Source: CAD feature listing. Evaluate the final solid. Frame: model axes, mm. Face numbers are marked on the shaded views. A direction names the side the tool comes from. Round coordinates to 2 decimals unless told otherwise and drop trailing zeros. Order: outer loops, then holes, each group sorted by start corner. A loop starts at its lowest first (then second) coordinate and runs counter-clockwise, first axis right, second up.
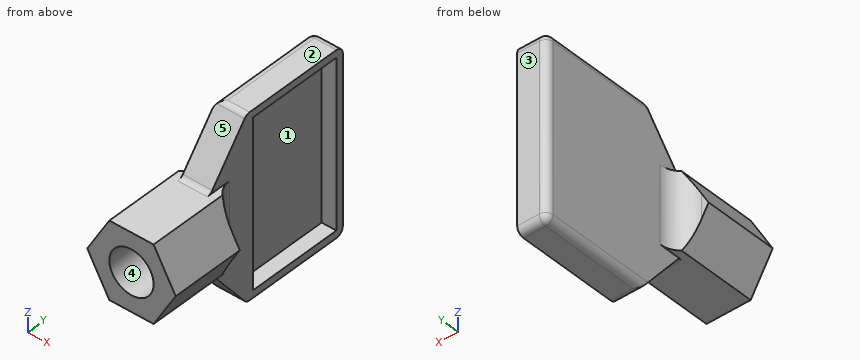
```python
from build123d import *

# Parameters (mm, degrees)
BOSS_EXTRUDE1_DEPTH      = 10
SKETCH2_R                = 3
CUT_EXTRUDE1_DEPTH       = 8
BOSS_EXTRUDE2_DEPTH      = 2
BOSS_EXTRUDE2_DEPTH_BACK = 2
SKETCH4_W                = 22.6
SKETCH4_H                = 13
CUT_EXTRUDE3_DEPTH       = 2
FILLET1_R                = 1
FILLET2_R                = 3


with BuildPart() as part:
    # Sketch1 → Boss-Extrude1 (new body)
    with BuildSketch(Plane(origin=(0, 0, 0), x_dir=(1, 0, 0), z_dir=(0, 1, 0))):
        Polygon((6, 0), (3, 5.196152423), (-3, 5.196152423), (-6, 0), (-3, -5.196152423), (3, -5.196152423), align=None)
    extrude(amount=BOSS_EXTRUDE1_DEPTH)

    # Sketch2 → Cut-Extrude1 (cut)
    with BuildSketch(Plane.XZ):
        with Locations(Location((0, 0, 0), (0, 0, 270))):
            Circle(SKETCH2_R)
    extrude(amount=-CUT_EXTRUDE1_DEPTH, mode=Mode.SUBTRACT)

    # Sketch3 → Boss-Extrude2 (add, two sides: drawn at the far end of the back side and taken through both)
    with BuildSketch(Plane(origin=(0, 0, 0), x_dir=(0, 0, -1), z_dir=(1, 0, 0)).offset(-BOSS_EXTRUDE2_DEPTH_BACK)):
        Polygon((0, 10), (5.196152423, 10), (12.3, 15.651732035), (12.3, 30.651732035), (0, 30.651732035), align=None)
        Polygon((-5.196152423, 10), (0, 10), (0, 30.651732035), (-12.3, 30.651732035), (-12.3, 15.651732035), align=None)
    extrude(amount=BOSS_EXTRUDE2_DEPTH + BOSS_EXTRUDE2_DEPTH_BACK)

    # Sketch4 → Cut-Extrude3 (cut)
    with BuildSketch(Plane(origin=(2, 0, 0), x_dir=(0, 0, -1), z_dir=(1, 0, 0))):
        with Locations((0, 23.151732035)):
            Rectangle(SKETCH4_W, SKETCH4_H)
    extrude(amount=-CUT_EXTRUDE3_DEPTH, mode=Mode.SUBTRACT)

    # Fillet1
    fillet1_edges = [part.edges().sort_by_distance(p)[0] for p in [
        (0, 30.651732035, 12.3),
        (-2, 30.651732035, 0),
        (0, 30.651732035, -12.3),
        (0, 15.651732035, -12.3),
        (0, 10, -5.196152423),
        (0, 10, 5.196152423),
        (0, 15.651732035, 12.3),
        (-2, 23.151732035, 12.3),
        (-2, 23.151732035, -12.3),
    ]]
    fillet(fillet1_edges, radius=FILLET1_R)

    # Fillet2
    fillet2_edges = [part.edges().sort_by_distance(p)[0] for p in [
        (-2, 10, 0),
        (2, 10, 0),
    ]]
    fillet(fillet2_edges, radius=FILLET2_R)


solid = part.part
```
1. Section D-D on x = -0.5. Return loops of the section in (y, z), plus the area to 3 significant figures.
2. First-contact query: pin 1 (8 mm diameter, centred on y = 14, z = -4, fed in from +X); pin 2 (5 mm diameter, centred on y = 9, z = 4, fed in from -X); pin 3 (1.8 mm diameter, centred on x = 0, y = 9.5, fed in from -Z). Flat tips, straight axial feed; report the tip coordinate or a pass-through.
3. Pull-direction query (Z, two-part tool) for the marked faces 3, 4 and 5; classes: released by +Z, released by -Z, zero draft, split by the parting line, or undercut.
4. Line query: line 1 along X through (y, z) = (28, 3.75); line 2 along Z through (x, y) = (1.5, 6.5); line 3 along Z through (x, y) = (0.5, 4.5). Output: solid intervals per line, ascending.
5. Section C-C on z = 7.5. Return loops of the section in (x, y), plus the area to 3 significant figures.
6. Section B-B on y = 24. Return loops of the section in (x, z), plus the area to 3 significant figures.
7. Section A-A on y = 3. Return loops of the section in (x, z).
8. Access query for the marked faces 1 and 2. Directions: +Z, -Z, +X, -X, +Y, -Y. A direction counts if a zero-diameter tool reaches every point of the face in a straight line with its end or side. Return the directions, or none.
Result:
1. outline: (0, -5.2) - (9.52, -5.2) arc R1 cw to (10.3, -5.57) - (15.35, -11.92) arc R1 ccw to (16.13, -12.3) - (29.65, -12.3) arc R1 ccw to (30.65, -11.3) - (30.65, 11.3) arc R1 ccw to (29.65, 12.3) - (16.13, 12.3) arc R1 ccw to (15.35, 11.92) - (10.3, 5.57) arc R1 cw to (9.52, 5.2) - (0, 5.2) - (0, 2.96) - (8, 2.96) - (8, -2.96) - (0, -2.96) - close
1. area: 524 mm2
2. pin 1: stops at x = 4.22
2. pin 2: stops at x = -5.13
2. pin 3: stops at z = -5.7
3. face 3: zero draft
3. face 4: undercut
3. face 5: released by +Z
4. line 1: x = -2 to 0
4. line 2: z = -5.2 to -2.6, 2.6 to 5.2
4. line 3: z = -5.2 to -2.96, 2.96 to 5.2
5. outline: (-2, 11.83) - (2, 11.83) - (2, 16.65) - (0, 16.65) - (0, 29.65) - (2, 29.65) - (2, 30.65) - (-1, 30.65) arc R1 ccw to (-2, 29.65) - close
5. area: 49.1 mm2
6. outline: (-2, -11.3) arc R1 ccw to (-1, -12.3) - (2, -12.3) - (2, -11.3) - (0, -11.3) - (0, 11.3) - (2, 11.3) - (2, 12.3) - (-1, 12.3) arc R1 ccw to (-2, 11.3) - close
6. area: 52.8 mm2
7. outline: (-6, 0) - (-3, -5.2) - (3, -5.2) - (6, 0) - (3, 5.2) - (-3, 5.2) - close; hole circle Ø6 at (0, 0)
8. face 1: +X
8. face 2: +Z, +X, -X, +Y, -Y
